from build123d import *

# Parameters (mm, degrees)
EXTRUDE1_DEPTH      = 1.6
SKETCH2_W           = 3
SKETCH2_H           = 3.2
LPATTERN1_COUNT     = 3
LPATTERN1_PITCH     = 1
LPATTERN1_COL_COUNT = 2
LPATTERN1_COL_PITCH = 1


with BuildPart() as part:
    # Sketch1 → Extrude1 (new body, symmetric)
    with BuildSketch(Plane(origin=(0, 0, 0), x_dir=(1, 0, 0), z_dir=(0, 1, 0))):
        Polygon((0, 5.773502692), (-5, 2.886751346), (-5, -2.886751346), (0, -5.773502692), (5, -2.886751346), (5, 2.886751346), align=None)
    extrude(amount=EXTRUDE1_DEPTH, both=True)

    # Sketch4 → Cut-Revolve2 (revolve, cut)
    with BuildSketch(Plane(origin=(0, 0, 0), x_dir=(0, 0, -1), z_dir=(1, 0, 0))):
        Polygon((0, 1.6), (3, 1.6), (2.538023184, 1.384576673), (2.538023184, -1.384576673), (3, -1.6), (0, -1.6), align=None)
    revolve(axis=Axis((0, 1.6, 0), (0, 1, 0)), mode=Mode.SUBTRACT)


with BuildPart() as body_2:
    # Sketch2 → Revolve1 (revolve)
    with BuildSketch(Plane(origin=(0, 0, 0), x_dir=(0, 0, -1), z_dir=(1, 0, 0))):
        with Locations((1.5, 0)):
            Rectangle(SKETCH2_W, SKETCH2_H)
    revolve(axis=Axis((0, -4.6, 0), (0, 1, 0)))

    # Sketch3 → Cut-Revolve1 (revolve, cut)
    with BuildSketch(Plane(origin=(0, 0, 0), x_dir=(0, 0, -1), z_dir=(1, 0, 0))):
        Polygon((3.020549873, 1.47670076), (3.164398987, 0.613606076), (2.579122931, 0.832870615), (2.538023184, 1.079469096), align=None)
    cut_revolve1 = revolve(axis=Axis((0, 1.6, 0.178376498), (0, -0.986393924, -0.164398987)), mode=Mode.SUBTRACT)

    # LPattern1: Cut-Revolve1 ×3
    with Locations(*[(0, -i * LPATTERN1_PITCH, 0) for i in range(1, LPATTERN1_COUNT)]):
        add(cut_revolve1, mode=Mode.SUBTRACT)

    # LPattern1 col: Cut-Revolve1 ×2
    with Locations(*[(0, i * LPATTERN1_COL_PITCH, 0) for i in range(1, LPATTERN1_COL_COUNT)]):
        add(cut_revolve1, mode=Mode.SUBTRACT)


with BuildPart() as part_1:
    add(part.part)

    # Combine1: cut body 2
    add(body_2.part, mode=Mode.SUBTRACT)

    # Sketch5 → Cut-Revolve3 (revolve, cut)
    with BuildSketch(Plane(origin=(0, 0, 0), x_dir=(0, 0, -1), z_dir=(1, 0, 0))):
        Polygon((0, -1.6), (5, -1.6), (5.773502692, -1.239309771), (5.773502692, 1.239309771), (5, 1.6), (0, 1.6), (0, 2.87), (7.043502692, 2.87), (7.043502692, -2.87), (0, -2.87), align=None)
    revolve(axis=Axis((0, -1.6, 0), (0, 1, 0)), mode=Mode.SUBTRACT)


solid = part_1.part
Design review of the part built by this model. Coordinates are the model's own, in mm. A direction names the side the tool comes from. Round coordinates to 2 decimals unless told otherwise and drop trailing zeros. Use a Markdown table: item, result. Add a question column.
1. For faces 1 (the face through (-2.535, 0.022, 4.31)), 2 (the face through (-0.11, -0.81, -2.67)), 3 (the face through (-2.735, -1.506, 0.597)), list the 3-axis set-ups (+Z, -Z, +X, -X, +Y, -Y) from which the entire face can be reached by the end or side of a thin tool; tool diameter is ignored.
2. Mouldability with a two-part tool opening along Z and no side actions: class faces 4 (the face through (5, 0, 0)), 5 (the face through (2.79, 1.5, -0.03)), 6 (the face through (0.01, -1.51, -5.19)) as +Z half, -Z half, draft (parallel to the pull), parting line (faces both ways), or undercut.
3. Wall thickness on probe 1 along X at (y, z) = (1.15, 0.25); probe 2 along X at (y, z) = (-1.05, 2); probe 3 along Z at (x, y) = (-3.5, 0.65): over which ranges is each line inside the solid? List them lowest first.
4. Clearance check with flat-ended pins moving along their axes: pin 1 (5 mm diameter, centred on x = 0, z = 0, fed in from -Y); pin 2 (1 mm diameter, centred on y = 0.5, z = 3.5, fed in from +X). State where each tip first meets the part, or that it passes through.
Output:
| question | item | result |
|---|---|---|
| 1 | face 1 | +Z, -X, +Y, -Y |
| 1 | face 2 | none |
| 1 | face 3 | -Y |
| 2 | face 4 | draft |
| 2 | face 5 | undercut |
| 2 | face 6 | -Z half |
| 3 | probe 1 | x = -5 to -2.94, 2.94 to 5 |
| 3 | probe 2 | x = -5 to -1.89, 1.89 to 5 |
| 3 | probe 3 | z = -3.75 to 3.75 |
| 4 | pin 1 | passes through |
| 4 | pin 2 | stops at x = 4.8 |
